from build123d import *

# Parameters (mm, degrees)
F1_DEPTH       = 10
F2_R           = 10
F3_R           = 5
F4_DEPTH       = 25
F6_ANGLE       = 180
F8_DEPTH       = 45
F9_R           = 10.5
F10_DEPTH      = 50
F10_DEPTH_BACK = 50
F11_W          = 14
F11_H          = 25.2948729652
F12_DEPTH      = 50


with BuildPart() as f1:
    # F0 (on Top) → F1 (new body)
    with BuildSketch(Plane.XY):
        with BuildLine():
            Line((-32.9545475543, 0), (-55, 0))
            Line((-55, 0), (-55, -26))
            Line((-55, -26), (-20.2485111676, -26))
            ThreePointArc((-20.2485111676, -26), (-29.6081300379, -14.4693068308), (-32.9545475543, 0))
        make_face()
        with BuildLine():
            Line((32.9545475543, 0), (-32.9545475543, 0))
            ThreePointArc((-32.9545475543, 0), (-29.6081300379, -14.4693068308), (-20.2485111676, -26))
            Line((-20.2485111676, -26), (20.2485111676, -26))
            ThreePointArc((20.2485111676, -26), (29.6081300379, -14.4693068308), (32.9545475543, 0))
        make_face()
        with BuildLine():
            Line((55, 0), (32.9545475543, 0))
            ThreePointArc((32.9545475543, 0), (29.6081300379, -14.4693068308), (20.2485111676, -26))
            Line((20.2485111676, -26), (55, -26))
            Line((55, -26), (55, 0))
        make_face()
        with BuildLine():
            Line((20.2485111676, -26), (-20.2485111676, -26))
            ThreePointArc((-20.2485111676, -26), (0, -32.9545475543), (20.2485111676, -26))
        make_face()
    extrude(amount=-F1_DEPTH)

    # F2
    f2_edges = [f1.edges().sort_by_distance(p)[0] for p in [
        (-55, -26, -5),
        (55, -26, -5),
    ]]
    fillet(f2_edges, radius=F2_R)

    # F3 (on Top) → F4 (cut)
    with BuildSketch(Plane.XY):
        with Locations((-45, -16.2500012666)):
            Circle(F3_R)
        with Locations((45, -16.2500012666)):
            Circle(F3_R)
    extrude(amount=-F4_DEPTH, mode=Mode.SUBTRACT)

    # F5 (on Front) → F6 (revolve)
    with BuildSketch(Plane.XZ):
        with BuildLine():
            Line((0, 9.8314080073), (0, 0))
            Line((0, 0), (24.3154959095, 0))
            ThreePointArc((24.3154959095, 0), (12.8138743622, 6.5384663753), (0, 9.8314080073))
        make_face()
    revolve(axis=Axis((0, 0, 4.9157040036), (0, 0, -1)), revolution_arc=F6_ANGLE)

    # F7 (on Top) → F8 (join)
    with BuildSketch(Plane.XY):
        with BuildLine():
            ThreePointArc((-14.3181821331, 0), (0, -14.3181821331), (14.3181821331, 0))
            Line((14.3181821331, 0), (-14.3181821331, 0))
        make_face()
    extrude(amount=F8_DEPTH)

    # F9 (on Top) → F10 (cut, two sides)
    with BuildSketch(Plane.XY) as f10_sk:
        Circle(F9_R)
    extrude(amount=-F10_DEPTH, mode=Mode.SUBTRACT)
    extrude(f10_sk.sketch, amount=F10_DEPTH_BACK, mode=Mode.SUBTRACT)

    # F11 (on Front) → F12 (cut)
    with BuildSketch(Plane.XZ):
        with Locations((0, -11.0227272962)):
            Rectangle(F11_W, F11_H)
    extrude(amount=F12_DEPTH, mode=Mode.SUBTRACT)


solid = f1.part
Can you work these out from the model? Positions are in its coordinate system, mm. A direction names the side the tool comes from. Give positions to 0.01 mm unless a question says otherwise; leave off trailing zeros. Loops run counter-clockwise (first coordinate to the right, second up) from the corner with the lowest first, then second, coordinate; pieces in that order, holes last. Notation, with made-up numbers: (47, 40.25) - (102, 40.25) arc R19 ccw to (102, 44.25) - close; hole circle Ø3 at (84.5, 64). An arc over 180 degrees is marked (long way). One line per item, written item: value.
(1) On a 3-axis mill with a long thin cutter (end or side, diameter ignored), from which of +Z, -Z, +X, -X, +Y, -Y can I reach the whole of each face in a straight line? I mean faces 1 (the face through (-31, -12, 0)), 2 (the face through (31, -12, 0)), 3 (the face through (-7, -20, -4)), 4 (the face through (32, -26, -5)). Say none if no direction works.
Verdict:
face 1: +Z, -X, -Y
face 2: +Z, +X, -Y
face 3: -Z, +Y, -Y
face 4: +Z, -Z, +X, -Y
(2) If we mould it in two halves opening along X, with no side actions, what happens to faces 5 (the face through (7, -20, -4)), 6 (the face through (-52.15, -22.99, -5.07)), 7 (the face through (-33, -26, -5))? For each: released by +X, released by -X, zero draft, split by the parting line, or undercut.
Verdict:
face 5: undercut
face 6: released by -X
face 7: zero draft
(3) If we section it at B-B, the plane z = 40: List the corners of the cut face in (x, y) for me.
Verdict:
outline: (-14.32, 0) arc R14.32 ccw to (14.32, 0) - (10.5, 0) arc R10.5 cw to (-10.5, 0) - close
(4) I need wall thicknesses on line 1 along Y through (x, z) = (-45, -3.75); line 2 along X through (y, z) = (-10.5, -5.5); line 3 along Y through (x, z) = (-0.5, 28). Which ranges of each line are inside material? Lowest first, please.
Verdict:
line 1: -26 to -21.25, -11.25 to 0
line 2: -55 to -7, 7 to 55
line 3: -14.31 to -10.49
(5) I'm going to push flat-ended pins straight in: pin 1 (4 mm diameter, centred on x = -17, y = -17.5, fed in from +Z); pin 2 (5 mm diameter, centred on y = -18.5, z = 13.5, fed in from +X); pin 3 (5 mm diameter, centred on x = -32, z = -4.5, fed in from -Y); pin 4 (3.5 mm diameter, centred on y = -24.5, z = -1.5, fed in from +X). Where does each tip first touch, or does it pass through?
Verdict:
pin 1: z = 1.39
pin 2: through
pin 3: y = -26
pin 4: x = 52.38
(6) If we section it at A-A, the plane z = -4: List the corners of the cut face in (x, y) for me.
Verdict:
outline: (-55, -16) arc R10 ccw to (-45, -26) - (-20.25, -26) arc R32.95 ccw to (-7, -32.2) - (-7, -7.83) arc R10.5 cw to (-10.5, 0) - (-55, 0) - close; (7, -32.2) arc R32.95 ccw to (20.25, -26) - (45, -26) arc R10 ccw to (55, -16) - (55, 0) - (10.5, 0) arc R10.5 cw to (7, -7.83) - close; hole circle Ø10 at (-45, -16.25); hole circle Ø10 at (45, -16.25)
